The model under review builds one solid part; all positions refer to its coordinate system, in mm. A direction names the side the tool comes from. Round coordinates to 2 decimals unless told otherwise and drop trailing zeros. Order: outer loops, then holes, each group sorted by start corner. A loop starts at its lowest first (then second) coordinate and runs counter-clockwise, first axis right, second up. Notation, with made-up numbers: (62, 39.25) - (103, 39.25) arc R26 ccw to (103, 78.25) - close; hole circle Ø2 at (45, 19.25). An arc over 180 degrees is marked (long way). One line per question, with ' | ' between items. Start each with the question number.
Item 1: Add section B-B on z = -46.5. State the section outline as (x, y) points, and give its area (3 significant figures).
Item 2: For L1, parallel to Z at x = -10, y = 6.7; L2, parallel to Z at x = 13.9, y = 8.05; L3, parallel to Z at x = 13.9, y = 9.1, list the stretches that pass through material, from the lowest coordinate up. Write a range as [from, to].
Item 3: Tool access review of faces 5 (the face through (11.28, 7.78, -84.67)), 6 (the face through (11.03, 7.288, -100.637)), 7 (the face through (16, 5.5, -49)), 8 (the face through (-14, 21, -5)): name each direction out of +Z, -Z, +X, -X, +Y, -Y from which nothing blocks a thin tool from reaching the whole face with its end or side.
Item 4: Draft analysis for pull direction X (two halves, no side actions). For faces 1 (the face through (7, 5, -76)), 2 (the face through (-6.5, 7.29, -32.79)), 3 (the face through (-15, 12, -6)), 4 (the face through (-19, 5, -123)), state which applies: +X half, -X half, draft (parallel to the pull), parting line (faces both ways), or undercut.
Item 5: Insertion check: pin 1 Ø23 at (x, z) = (-2, -112.5) entering from +Y; pin 2 Ø5 at (x, y) = (7.5, 10) entering from +Z; pin 3 Ø5 at (x, y) = (-13, 19) entering from -Z. Each pin has a flat end and moves straight along its axis. Give the tip position at first contact, or say it passes through.
Item 6: Add section A-A on z = -112.5. State the section outline as (x, y) points, and give its area (3 significant figures).
Item 7: Add section C-C on y = 7.5. State how many separate pieces and enclosed holes the cut face has, and give its area (3 significant figures).
from build123d import *

# Parameters (mm, degrees)
EXTRUDE_1_DEPTH           = 20
SKETCH_2_W                = 29
SKETCH_2_H                = 5
CUT_EXTRUDE_1_DEPTH       = 18
FILLET_1_R                = 5
CHAMFER_1_SIZE            = 10
SKETCH_3_R                = 10
CUT_EXTRUDE_2_DEPTH       = 128.863208156
HOLE_WIZARD_1_D           = 5.5
HOLE_WIZARD_1_CBORE_D     = 9.5
HOLE_WIZARD_1_CBORE_DEPTH = 5.5
HOLE_WIZARD_2_D           = 5.5
HOLE_WIZARD_2_DEPTH       = 31
HOLE_WIZARD_2_CBORE_D     = 9.5
HOLE_WIZARD_2_CBORE_DEPTH = 5.5
SKETCH_9_R                = 7.25
CUT_EXTRUDE_3_DEPTH       = 128.863208156
FILLET_2_R                = 5


with BuildPart() as part:
    # 草图1 → 凸台-拉伸1 (new, symmetric)
    with BuildSketch(Plane(origin=(0, 0, 0), x_dir=(0, 0, -1), z_dir=(1, 0, 0))):
        Polygon((0, 28), (0, 0), (125, 0), (125, 10), (5, 10), (5, 28), align=None)
    extrude(amount=EXTRUDE_1_DEPTH, both=True)

    # 草图2 → 切除-拉伸1 (cut)
    with BuildSketch(Plane(origin=(0, 28, 0), x_dir=(1, 0, 0), z_dir=(0, 1, 0))):
        with Locations((5.5, 2.5)):
            Rectangle(SKETCH_2_W, SKETCH_2_H)
    extrude(amount=-CUT_EXTRUDE_1_DEPTH, mode=Mode.SUBTRACT)

    # 圆角1
    fillet_1_edges = [part.edges().sort_by_distance(p)[0] for p in [
        (-14.5, 10, -5),
    ]]
    fillet(fillet_1_edges, radius=FILLET_1_R)

    # 倒角1
    chamfer_1_edges = [part.edges().sort_by_distance(p)[0] for p in [
        (5.5, 10, 0),
    ]]
    chamfer(chamfer_1_edges, length=CHAMFER_1_SIZE - 0.0001)  # a hair under: the kernel refuses the full size

    # 草图3 → 切除-拉伸2 (cut, through all)
    with BuildSketch(Plane(origin=(0, 10, 0), x_dir=(1, 0, 0), z_dir=(0, 1, 0))):
        with Locations(Location((7, 66, 0), (0, 0, 270))):
            Circle(SKETCH_3_R)
    extrude(amount=-CUT_EXTRUDE_2_DEPTH, mode=Mode.SUBTRACT)

    # 孔1 (through all)
    with Locations(Plane.XZ):
        with Locations((13.9, -46.5), (0.1, -46.5), (0.1, -85.5), (13.9, -85.5)):
            CounterBoreHole(HOLE_WIZARD_1_D / 2, HOLE_WIZARD_1_CBORE_D / 2, HOLE_WIZARD_1_CBORE_DEPTH)

    # 孔2
    with Locations(Plane(origin=(0, 10, 0), x_dir=(-1, 0, 0), z_dir=(0, 1, 0))):
        with Locations((-10, -96), (10, -96), (10, -36), (-10, -36)):
            CounterBoreHole(HOLE_WIZARD_2_D / 2, HOLE_WIZARD_2_CBORE_D / 2, HOLE_WIZARD_2_CBORE_DEPTH, depth=HOLE_WIZARD_2_DEPTH)

    # 草图9 → 切除-拉伸3 (cut, through all)
    with BuildSketch(Plane(origin=(0, 10, 0), x_dir=(1, 0, 0), z_dir=(0, 1, 0))):
        with Locations(Location((-2, 112.5, 0), (0, 0, 270))):
            Circle(SKETCH_9_R)
    extrude(amount=-CUT_EXTRUDE_3_DEPTH, mode=Mode.SUBTRACT)

    # 圆角2
    fillet_2_edges = [part.edges().sort_by_distance(p)[0] for p in [
        (20, 5, -125),
        (-20, 5, -125),
    ]]
    fillet(fillet_2_edges, radius=FILLET_2_R)


solid = part.part
Determined:
1) outline: (-20, 0) - (-4.65, 0) - (-4.65, 5.5) - (-2.65, 5.5) - (-2.65, 10) - (-20, 10) - close; (2.85, 5.5) - (4.85, 5.5) - (4.85, 0) - (9.15, 0) - (9.15, 5.5) - (11.15, 5.5) - (11.15, 10) - (2.85, 10) - close; (16.65, 5.5) - (18.65, 5.5) - (18.65, 0) - (20, 0) - (20, 10) - (16.65, 10) - close | area: 246 mm2
2) L1: [-125, -100.75], [-91.25, -40.75], [-31.25, 0] | L2: [-125, -98.71], [-93.29, -88.25], [-82.75, -73.24], [-58.76, -49.25], [-43.75, -38.71], [-33.29, -8.05] | L3: [-125, -98.71], [-93.29, -88.25], [-82.75, -73.24], [-58.76, -49.25], [-43.75, -38.71], [-33.29, -9.1]
3) face 5: +Y, -Y | face 6: +Y | face 7: -Y | face 8: -Z, +X, -X, +Y
4) face 1: undercut | face 2: undercut | face 3: draft | face 4: -X half
5) pin 1: y = 10 | pin 2: z = -7.5 | pin 3: z = -5
6) outline: (-20, 0) - (-9.25, 0) - (-9.25, 10) - (-20, 10) - close; (5.25, 0) - (20, 0) - (20, 10) - (5.25, 10) - close | area: 255 mm2
7) separate pieces: 1 | enclosed holes: 10 | area: 3,910 mm2
